Design review of the part built by this model. Coordinates are the model's own, in mm. Face numbers are marked on the shaded views. Round coordinates to 2 decimals unless told otherwise and drop trailing zeros. Write item = value, one per line. Start each with the question number.
Item 1: Mouldability with a two-part tool opening along X and no side actions: class the marked faces 1, 2 and 3 as released by +X, released by -X, zero draft, split by the parting line, or undercut.
Item 2: To check wall thickness, follow L1, parallel to X at y = 0.2, z = 0; L2, parallel to Z at x = -4.5, y = -0.7; L3, parallel to Z at x = 3.75, y = 0.2. State the ranges of each line that lie inside material, in increasing order.
Item 3: For pin 1 Ø8 at (x, z) = (-1, -3) entering from -Y; pin 2 Ø1 at (x, z) = (5, -1.5) entering from +Y; pin 3 Ø5 at (x, z) = (-2.5, -2) entering from -Y, all flat-tipped, find the tip position at first contact; note any pin that passes through.
from build123d import *

# Parameters (mm, degrees)
SKETCH1_R           = 5.55625
BOSS_EXTRUDE1_DEPTH = 1
CHAMFER1_SIZE       = 0.25


with BuildPart() as part:
    # Sketch1 → Boss-Extrude1 (new, symmetric)
    with BuildSketch(Plane(origin=(0, 0, 0), x_dir=(1, 0, 0), z_dir=(0, 1, 0))):
        Polygon((0, 8.25), (-7.144709581, 4.125), (-7.144709581, -4.125), (0, -8.25), (7.144709581, -4.125), (7.144709581, 4.125), align=None)
        with Locations(Location((0, 0, 0), (0, 0, 270))):
            Circle(SKETCH1_R, mode=Mode.SUBTRACT)
    extrude(amount=BOSS_EXTRUDE1_DEPTH, both=True)

    # Sketch4 → Cut-Revolve1 (revolve, cut)
    with BuildSketch(Plane.XY):
        Polygon((-7.144709581, 1), (-8.25, 0.5), (-8.644709581, 0.5), (-8.644709581, 2), (-7.144709581, 2), align=None)
        Polygon((-7.144709581, -2), (-7.144709581, -1), (-8.25, -0.5), (-8.644709581, -0.5), (-8.644709581, -2), align=None)
    revolve(axis=Axis((0, 1, 0), (0, -1, 0)), mode=Mode.SUBTRACT)

    # Chamfer1
    chamfer1_edges = [part.edges().sort_by_distance(p)[0] for p in [
        (0, -1, -5.55625),
        (0, 1, -5.55625),
    ]]
    chamfer(chamfer1_edges, length=CHAMFER1_SIZE)


solid = part.part
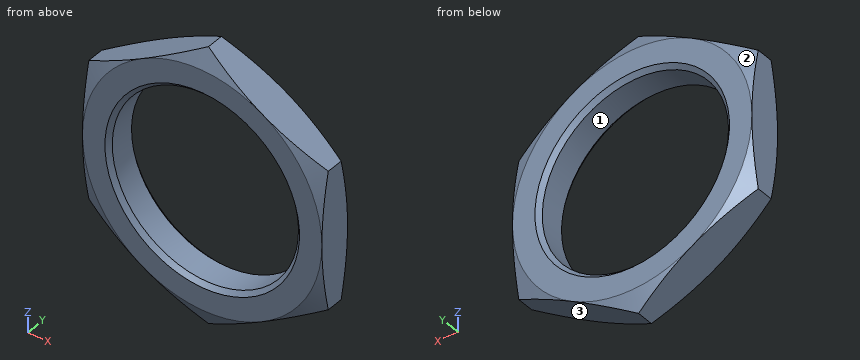
Result set:
q1.face_1 = undercut
q1.face_2 = released by -X
q1.face_3 = released by +X
q2.L1 = -7.14 to -5.56, 5.56 to 7.14
q2.L2 = -5.65 to -3.26, 3.26 to 5.65
q2.L3 = -6.08 to -4.1, 4.1 to 6.08
q3.pin_1 = -1
q3.pin_2 = 0.91
q3.pin_3 = -0.9
